Read the model definition and answer for the solid it produces. Units are mm, in the model's axes. Coordinates: 2 decimals unless noted, no trailing zeros. Write each loop counter-clockwise with the first axis right and the second up, starting at its lowest first coordinate (ties: lowest second). Pieces come first, ordered by that corner, then holes. Notation, with made-up numbers: (85.5, 10.25) -> (108.5, 10.25) arc R34 ccw to (108.5, 45.25) -> close; hole circle Ø2 at (-24, 17). An arc over 180 degrees is marked (long way). Answer as a JSON object with one key per item and string values. Group by question number.
(1) Find section A-A (x = -11). Give the vertices of the cut face in (y, z).
(2) Find section B-B (z = -3.5). Give the vertices of the cut face in (x, y), then the cut area to 3 significant figures.
(3) For a pull along Z with two mould halves and no side action, classify faces 1 (the face through (122.13, 2.46, 114.98)), 2 (the face through (-20.49, 2.46, -23.69)), 3 (the face through (-35, 0, 2)), 4 (the face through (-120.51, 2.46, -106.82)) as +Z half, -Z half, draft (parallel to the pull), parting line (faces both ways), or undercut.
(4) Straight lines are drawn through the part: L1, parallel to Z at x = -20.5, y = 1.5; L2, parallel to X at y = 3.75, z = 28.5; L3, parallel to Z at x = -13.5, y = 3.6. For each, find the intervals that lie inside material, in ascending order.
(5) Find section C-C (y = 1.3). Give the vertices of the cut face in (x, z).
(6) Find section D-D (z = 122). Give the vertices of the cut face in (x, y), then the cut area to 3 significant figures.
from build123d import *

# Parameters (mm, degrees)
SKETCH_1_R      = 35
EXTRUDE_1_DEPTH = 5


with BuildPart() as part:
    # Эскиз1 → Вытянуть1 (new body)
    with BuildSketch(Plane(origin=(0, 0, 0), x_dir=(1, 0, 0), z_dir=(0, 1, 0))):
        Polygon((-151.693051502, 77.916478726), (-151.693051502, -86.083521274), (-90.193051502, -143.083521274), (91.806948498, -143.083521274), (153.306948498, -86.083521274), (153.306948498, 77.916478726), (91.806948498, 134.916478726), (-90.193051502, 134.916478726), align=None)
        with Locations(Location((0.806948498, -4.083521274, 0), (0, 0, 270))):
            Circle(SKETCH_1_R, mode=Mode.SUBTRACT)
    extrude(amount=EXTRUDE_1_DEPTH)


solid = part.part
Results below:
{
 "1": {"outline": "(0, -134.92) -> (5, -134.92) -> (5, -28.86) -> (0, -28.86) -> close; (0, 37.03) -> (5, 37.03) -> (5, 143.08) -> (0, 143.08) -> close"},
 "2": {"outline": "(-151.69, 0) -> (-33.36, 0) -> (-33.36, 5) -> (-151.69, 5) -> close; (34.98, 0) -> (153.31, 0) -> (153.31, 5) -> (34.98, 5) -> close", "area": "1,180 mm2"},
 "3": {"face 1": "+Z half", "face 2": "undercut", "face 3": "draft", "face 4": "-Z half"},
 "4": {"L1": "z = -134.92 to -23.68, 31.85 to 143.08", "L2": "x = -151.69 to -24.27, 25.88 to 153.31", "L3": "z = -134.92 to -27.86, 36.03 to 143.08"},
 "5": {"outline": "(-151.69, -77.92) -> (-90.19, -134.92) -> (91.81, -134.92) -> (153.31, -77.92) -> (153.31, 86.08) -> (91.81, 143.08) -> (-90.19, 143.08) -> (-151.69, 86.08) -> close; hole circle Ø70 at (0.81, 4.08)"},
 "6": {"outline": "(-112.94, 0) -> (114.55, 0) -> (114.55, 5) -> (-112.94, 5) -> close", "area": "1,140 mm2"}
}
